Verification items for the finished model (mm, model axes). A direction names the side the tool comes from. Coordinates: 2 decimals unless noted, no trailing zeros. Order: outer loops, then holes, each group sorted by start corner. A loop starts at its lowest first (then second) coordinate and runs counter-clockwise, first axis right, second up. Notation, with made-up numbers: M -27,89 L 4,89 A20 cw 4,106 Z; hole C -22,-39.75 d3. An arc over 180 degrees is marked long. Return JSON: item names as keys, results as strings. Group by question number.
Q1. Section check B-B, the plane x = -24.75. Enter the section's corners in (y, z), then the cut area to 3 significant figures.
Q2. Access from +Z, -Z, +X, -X, +Y, -Y to the whole of each face (thin tool, end or side, straight path). Record for faces 1 (the face through (-37, 21.258, 1)), 2 (the face through (-32.831, 15, 1)), 3 (the face through (-29.824, 22.477, 4.493)).
Q3. Section check C-C, the plane y = 13. Enter the section's corners in (x, z), then the cut area to 3 significant figures.
Q4. Section check A-A, the plane z = 0.85. Enter the section's corners in (x, y), then the cut area to 3 significant figures.
Q5. Go/stop test with flat-tipped pins: pin 1 Ø0.6 at (y, z) = (26.5, 1) entering from +X; pin 2 Ø1 at (y, z) = (27, 4) entering from +X; pin 3 Ø1.5 at (y, z) = (26.5, 2) entering from +X. Record where each tip stops, or that it passes through.
Q6. Mould release check, pull along X, two halves, no side actions. Record for faces 4 (the face through (-28.94, 16.096, 4.493)), 5 (the face through (-27.178, 11.774, 2.465)), 6 (the face through (-36, 15, 0)), 7 (the face through (-23.941, 16.694, 4.493)): pulls with the +X half, pulls with the -X half, needs draft (parallel to the pull), parting line crosses it, or undercut.
Q7. Thickness scan on probe 1 along X at (y, z) = (16.5, 4.3) (3 decimals); probe 2 along Y at (x, z) = (-34.5, 4.45); probe 3 along X at (y, z) = (16.75, 4.45). Record the ranges inside material, lowest first.
Q8. Section check D-D, the plane z = 4.55. Count the separate pieces of the cut face and the enclosed holes in it, then the cut area to 3 significant figures.
from build123d import *

# Parameters (mm, degrees)
F0_R     = 9
F1_DEPTH = 4
F3_W     = 3
F3_H     = 3
F4_DEPTH = 2
F2_R     = 9
F2_R_2   = 8
F5_DEPTH = 1
F7_DEPTH = 1


# Not quite as in the source:
# - a feature names something its author has since deleted; it is built from what else it names


with BuildPart() as f1:
    # F0 (on Top) → F1 (new body)
    with BuildSketch(Plane.XY):
        with Locations((-31.3306450844, 19.7580661625)):
            Circle(F0_R)
    extrude(amount=F1_DEPTH)

    # F3 (on face) → F4 (cut)
    with BuildSketch(Plane(origin=(0, 0, 0), x_dir=(1, 0, 0), z_dir=(0, 0, -1))):
        with BuildLine():
            ThreePointArc((-32.8306450844, -28.6321858371), (-32.0832814269, -28.7265408676), (-31.3306450844, -28.7580661625))
            ThreePointArc((-31.3306450844, -28.7580661625), (-30.5780087419, -28.7265408676), (-29.8306450844, -28.6321858371))
            Line((-29.8306450844, -28.6321858371), (-29.8306450844, -21.2580661625))
            Line((-29.8306450844, -21.2580661625), (-32.8306450844, -21.2580661625))
            Line((-32.8306450844, -21.2580661625), (-32.8306450844, -28.6321858371))
        make_face()
        with BuildLine():
            ThreePointArc((-40.204764759, -18.2580661625), (-40.2991197895, -19.0054298199), (-40.3306450844, -19.7580661625))
            ThreePointArc((-40.3306450844, -19.7580661625), (-40.2991197895, -20.510702505), (-40.204764759, -21.2580661625))
            Line((-40.204764759, -21.2580661625), (-32.8306450844, -21.2580661625))
            Line((-32.8306450844, -21.2580661625), (-32.8306450844, -18.2580661625))
            Line((-32.8306450844, -18.2580661625), (-40.204764759, -18.2580661625))
        make_face()
        with Locations((-31.3306450844, -19.7580661625)):
            Rectangle(F3_W, F3_H)
        with BuildLine():
            Line((-29.8306450844, -18.2580661625), (-29.8306450844, -21.2580661625))
            Line((-29.8306450844, -21.2580661625), (-22.4565254097, -21.2580661625))
            ThreePointArc((-22.4565254097, -21.2580661625), (-22.3621703793, -20.510702505), (-22.3306450844, -19.7580661625))
            ThreePointArc((-22.3306450844, -19.7580661625), (-22.3621703793, -19.0054298199), (-22.4565254097, -18.2580661625))
            Line((-22.4565254097, -18.2580661625), (-29.8306450844, -18.2580661625))
        make_face()
        with BuildLine():
            Line((-32.8306450844, -10.8839464878), (-32.8306450844, -18.2580661625))
            Line((-32.8306450844, -18.2580661625), (-29.8306450844, -18.2580661625))
            Line((-29.8306450844, -18.2580661625), (-29.8306450844, -10.8839464878))
            ThreePointArc((-29.8306450844, -10.8839464878), (-30.5780087419, -10.7895914574), (-31.3306450844, -10.7580661625))
            ThreePointArc((-31.3306450844, -10.7580661625), (-32.0832814269, -10.7895914574), (-32.8306450844, -10.8839464878))
        make_face()
    extrude(amount=-F4_DEPTH, mode=Mode.SUBTRACT)

    # F2 (on face) → F5 (join)
    with BuildSketch(Plane.XY.offset(4)):
        with Locations((-31.3306450844, 19.7580661625)):
            Circle(F2_R)
        with Locations((-31.3306450844, 19.7580661625)):
            Circle(F2_R_2, mode=Mode.SUBTRACT)
    extrude(amount=F5_DEPTH)

    # F6 (on face) → F7 (join)
    with BuildSketch(Plane.XY.offset(4)):
        Polygon((-33.5311048114, 20.2471387647), (-33.3884463109, 19.0475286451), (-36.4782309787, 18.7233090579), (-36.6460120564, 18.6325285146), (-36.5527999544, 18.4574668773), (-36.1151093936, 18.1818667), (-35.5996001325, 18.1688972107), (-31.940004334, 18.7654525459), (-27.1472810179, 18.9729526111), (-26.8433067742, 18.9470136325), (-26.5182754911, 18.9599831218), (-26.3042936222, 18.9607948177), (-26.1681286891, 19.0734676237), (-26.1713637091, 19.2331364476), (-26.3172925208, 19.4268553276), (-27.0038225852, 19.8199867228), (-27.5623046758, 19.8775230241), (-28.8218450116, 19.6546301455), (-30.3473039921, 19.4138858383), (-30.18602354, 20.0915166568), (-30.0238608098, 20.6159310458), (-29.880402377, 20.9895817386), (-29.7734114426, 21.2100336476), (-29.8042323605, 21.3373169803), (-29.9225752742, 21.5375353096), (-30.1624961218, 21.6996392213), (-29.3754451629, 21.8673897134), (-28.780495574, 21.9970846065), (-28.3971162937, 22.088665082), (-28.2398943213, 22.1405430392), (-28.1782524855, 22.3642887867), (-28.3590018762, 22.5125703402), (-28.6807981392, 22.649558733), (-29.2765711877, 22.5985042354), (-30.3861830508, 22.3512898882), (-31.7138705535, 22.078960022), (-32.9734520623, 21.9006221917), (-32.9856098557, 22.6074446543), (-32.960482573, 23.0029993736), (-32.999385159, 23.3045032384), (-31.4617801489, 23.6870590591), (-30.3732429707, 24.0826137783), (-29.7652944833, 24.2577165886), (-29.1574048143, 24.3841764617), (-28.9807139033, 24.3874114817), (-28.8559009495, 24.4975786176), (-28.8615475299, 24.6426839697), (-28.956421844, 24.8250802796), (-29.338154205, 25.0698242479), (-29.860992257, 25.3405660134), (-30.2597819962, 25.4540269879), (-30.3861830508, 25.2530440175), (-30.6026352986, 24.9539517131), (-31.1318963358, 24.5729839931), (-31.9878296934, 24.1077292973), (-33.1874221675, 23.554129146), (-33.564325526, 23.7632878942), (-33.9655444712, 23.9335087652), (-34.1811556138, 23.9440372849), (-34.3189557025, 23.9075697866), (-34.4056660024, 23.7616409749), (-34.3319251918, 23.5671280446), (-34.0466140726, 22.9738253749), (-33.8164159306, 22.3512898882), (-33.7499509741, 21.8957990709), (-33.6534885593, 21.1954466483), align=None)
        Polygon((-31.2348405543, 19.2906962764), (-31.5663359955, 19.2615222777), (-32.7594584296, 19.1123702098), (-32.8794306171, 20.3597939252), (-32.9475130837, 21.4240155165), (-32.3266362799, 21.3794898775), (-31.491783489, 21.4726584538), (-31.189438519, 21.502655912), (-30.8368507473, 21.5861782468), (-30.8019713497, 21.3049079617), (-30.78820781, 20.8445116777), (-30.8093236679, 20.1960725034), (-30.875765097, 19.3490442736), align=None, mode=Mode.SUBTRACT)
        Polygon((-33.2968599535, 17.7190588557), (-33.4014158002, 17.5788295611), (-34.506992711, 16.59725979), (-35.8881580354, 15.5816534911), (-35.9829911765, 15.4219770208), (-35.8622190568, 15.3287649188), (-35.4999026976, 15.3879328466), (-34.9779175146, 15.5938112845), (-34.3051745173, 15.940721302), (-33.4889613235, 16.4213746931), (-32.8721312356, 16.846909225), (-32.4449733118, 17.0503566924), (-32.2763817145, 17.1662645184), (-32.2309973247, 17.4037443963), (-32.4352388425, 17.6704218003), (-32.7724279189, 18.0554362362), (-33.0869306823, 18.1818667), (-33.2644274074, 18.0910861567), (-33.2619982015, 17.9289881268), align=None)
        Polygon((-30.5726378404, 17.8665698862), (-30.4478248866, 17.7182471597), (-29.4719075777, 16.6815585296), (-28.392293173, 15.4941144379), (-28.1758409251, 15.2452784634), (-27.9383904565, 15.1147812853), (-27.8313407034, 15.1342343429), (-27.7016458104, 15.2412252774), (-27.6108887945, 15.5224832106), (-27.6627667517, 16.0841914985), (-27.9318615979, 16.5113435404), (-28.4684631895, 17.0130716164), (-29.2895112678, 17.5723359936), (-30.4121220294, 18.1688972107), (-30.5321118624, 18.1867427574), (-30.5742259411, 18.0684057255), align=None)
    extrude(amount=F7_DEPTH)


solid = f1.part
Numbers:
{
 "1": {"outline": "M 13.62,0 L 18.26,0 L 18.26,2 L 21.26,2 L 21.26,0 L 25.9,0 L 25.9,5 L 24.31,5 L 24.31,4 L 15.21,4 L 15.21,5 L 13.62,5 Z", "area": "46.3 mm2"},
 "2": {"face 1": "-Z, +X, -X", "face 2": "-Z, +Y, -Y", "face 3": "+Z"},
 "3": {"outline": "M -37.27,0 L -32.83,0 L -32.83,2 L -29.83,2 L -29.83,0 L -25.39,0 L -25.39,5 L -27.05,5 L -27.05,4 L -35.61,4 L -35.61,5 L -37.27,5 Z", "area": "44.9 mm2"},
 "4": {"outline": "M -40.2,18.26 A9 ccw -32.83,10.88 L -32.83,18.26 Z; M -40.2,21.26 L -32.83,21.26 L -32.83,28.63 A9 ccw Z; M -29.83,10.88 A9 ccw -22.46,18.26 L -29.83,18.26 Z; M -29.83,21.26 L -22.46,21.26 A9 ccw -29.83,28.63 Z", "area": "156 mm2"},
 "5": {"pin 1": "stops at x = -25.05", "pin 2": "stops at x = -25.37", "pin 3": "stops at x = -24.62"},
 "6": {"face 4": "undercut", "face 5": "parting line crosses it", "face 6": "needs draft", "face 7": "undercut"},
 "7": {"probe 1": "x = -39.72 to -38.637, -34.639 to -33.375, -29.307 to -27.925, -24.024 to -22.941", "probe 2": "y = 11.33 to 12.41, 15.84 to 16.6, 18.35 to 18.93, 27.1 to 28.18", "probe 3": "x = -39.81 to -38.74, -34.33 to -33.01, -29.54 to -28.19, -23.92 to -22.85"},
 "8": {"separate pieces": "4", "enclosed holes": "2", "area": "77.6 mm2"}
}
